Design review of the part built by this model. Coordinates are the model's own, in mm. A direction names the side the tool comes from. Give positions to 0.01 mm unless a question says otherwise; leave off trailing zeros. Loops run counter-clockwise (first coordinate to the right, second up) from the corner with the lowest first, then second, coordinate; pieces in that order, holes last. Notation, with made-up numbers: (0, 44.5) - (40, 44.5) arc R28 ccw to (40, 70.5) - close; hole circle Ø5 at (12, 43). An arc over 180 degrees is marked (long way). One line per item, written item: value. Start each with the question number.
```python
from build123d import *

# Parameters (mm, degrees)
SKETCH1_R                       = 13
BOSS_EXTRUDE1_DEPTH             = 28
SKETCH3_R                       = 24
BOSS_EXTRUDE2_DEPTH             = 1
SKETCH2_R                       = 10
CUT_EXTRUDE1_DEPTH              = 1
CUT_EXTRUDE1_DEPTH_BACK         = 30
SKETCH9_R                       = 13
BOSS_EXTRUDE3_DEPTH             = 17.5
CHAMFER2_SIZE                   = 0.5
CHAMFER3_SIZE                   = 0.5
CHAMFER4_SIZE                   = 0.5
SKETCH11_R                      = 10
CUT_EXTRUDE5_DEPTH              = 1
CUT_EXTRUDE5_DEPTH_BACK         = 46.5
CHAMFER5_SIZE                   = 0.5
SKETCH7_R                       = 2.5
WYTNIJ_WYCI_GNI_CIE1_DEPTH      = 28
WYTNIJ_WYCI_GNI_CIE1_DEPTH_BACK = 19.5
WYTNIJ_WYCI_GNI_CIE2_DEPTH      = 10
ZAOKR_GLENIE1_R                 = 4
ZAOKR_GLENIE2_R                 = 1


with BuildPart() as part:
    # Sketch1 → Boss-Extrude1 (new body)
    with BuildSketch(Plane(origin=(0, 0, 0), x_dir=(1, 0, 0), z_dir=(0, 1, 0))):
        Circle(SKETCH1_R)
    extrude(amount=-BOSS_EXTRUDE1_DEPTH)

    # Sketch3 → Boss-Extrude2 (add, symmetric)
    with BuildSketch(Plane(origin=(0, 0, 0), x_dir=(1, 0, 0), z_dir=(0, 1, 0))):
        Circle(SKETCH3_R)
    extrude(amount=BOSS_EXTRUDE2_DEPTH, both=True)

    # Sketch2 → Cut-Extrude1 (cut, two sides)
    with BuildSketch(Plane(origin=(0, -28, 0), x_dir=(-1, 0, 0), z_dir=(0, -1, 0))) as cut_extrude1_sk:
        Circle(SKETCH2_R)
    extrude(amount=CUT_EXTRUDE1_DEPTH, mode=Mode.SUBTRACT)
    extrude(cut_extrude1_sk.sketch, amount=-CUT_EXTRUDE1_DEPTH_BACK, mode=Mode.SUBTRACT)

    # Sketch9 → Boss-Extrude3 (add)
    with BuildSketch(Plane(origin=(0, 0, 0), x_dir=(1, 0, 0), z_dir=(0, 1, 0))):
        Circle(SKETCH9_R)
    extrude(amount=BOSS_EXTRUDE3_DEPTH)

    # Chamfer2
    chamfer2_edges = [part.edges().sort_by_distance(p)[0] for p in [
        (-24, -1, 0),
    ]]
    chamfer(chamfer2_edges, length=CHAMFER2_SIZE)

    # Chamfer3
    chamfer3_edges = [part.edges().sort_by_distance(p)[0] for p in [
        (-24, 1, 0),
    ]]
    chamfer(chamfer3_edges, length=CHAMFER3_SIZE)

    # Chamfer4
    chamfer4_edges = [part.edges().sort_by_distance(p)[0] for p in [
        (-13, -28, 0),
    ]]
    chamfer(chamfer4_edges, length=CHAMFER4_SIZE)

    # Sketch11 → Cut-Extrude5 (cut, two sides)
    with BuildSketch(Plane(origin=(0, 17.5, 0), x_dir=(1, 0, 0), z_dir=(0, 1, 0))) as cut_extrude5_sk:
        Circle(SKETCH11_R)
    extrude(amount=CUT_EXTRUDE5_DEPTH, mode=Mode.SUBTRACT)
    extrude(cut_extrude5_sk.sketch, amount=-CUT_EXTRUDE5_DEPTH_BACK, mode=Mode.SUBTRACT)

    # Chamfer5
    chamfer5_edges = [part.edges().sort_by_distance(p)[0] for p in [
        (-13, 17.5, 0),
    ]]
    chamfer(chamfer5_edges, length=CHAMFER5_SIZE)

    # Sketch7 → Wytnij-wyciągnięcie1 (cut, two sides)
    with BuildSketch(Plane.XZ.offset(1)) as wytnij_wyci_gni_cie1_sk:
        with Locations((0, 19)):
            Circle(SKETCH7_R)
        with Locations((3.299315376, -18.711347307)):
            Circle(SKETCH7_R)
        with Locations((-6.497936067, 17.852932618)):
            Circle(SKETCH7_R)
        with Locations((9.5, 16.454482672)):
            Circle(SKETCH7_R)
        with Locations((-19, 0)):
            Circle(SKETCH7_R)
        with Locations((-8.029746973, -17.219847954)):
            Circle(SKETCH7_R)
        with Locations((-12.212964584, 14.554844419)):
            Circle(SKETCH7_R)
        with Locations((-14.575405337, -12.230217242)):
            Circle(SKETCH7_R)
        with Locations((-16.454482672, 9.5)):
            Circle(SKETCH7_R)
    extrude(amount=WYTNIJ_WYCI_GNI_CIE1_DEPTH, mode=Mode.SUBTRACT)
    extrude(wytnij_wyci_gni_cie1_sk.sketch, amount=-WYTNIJ_WYCI_GNI_CIE1_DEPTH_BACK, mode=Mode.SUBTRACT)

    # Szkic1 → Wytnij-wyciągnięcie2 (cut)
    with BuildSketch(Plane(origin=(0, 1, 0), x_dir=(1, 0, 0), z_dir=(0, 1, 0))):
        with BuildLine():
            Line((13.831592317, -13.026398351), (17.289813207, -16.645190274))
            ThreePointArc((17.289813207, -16.645190274), (23.635386072, 4.167556264), (10.554119522, 21.554826863))
            Line((10.554119522, 21.554826863), (8.542154603, 16.971493592))
            ThreePointArc((8.542154603, 16.971493592), (18.711347307, 3.299315376), (13.831592317, -13.026398351))
        make_face()
    extrude(amount=-WYTNIJ_WYCI_GNI_CIE2_DEPTH, mode=Mode.SUBTRACT)

    # Zaokrąglenie1
    zaokr_glenie1_edges = [part.edges().sort_by_distance(p)[0] for p in [
        (13.831592317, 0, 13.026398351),
        (8.542154603, 0, -16.971493592),
    ]]
    fillet(zaokr_glenie1_edges, radius=ZAOKR_GLENIE1_R)

    # Zaokrąglenie2
    zaokr_glenie2_edges = [part.edges().sort_by_distance(p)[0] for p in [
        (10.554119522, 0, -21.554826863),
        (17.289813207, 0, 16.645190274),
    ]]
    fillet(zaokr_glenie2_edges, radius=ZAOKR_GLENIE2_R)


solid = part.part
```
(1) Draft analysis for pull direction X (two halves, no side actions). For faces 1 (the cylindrical face through (-10.316, -14.064, 7.91)), 2 (the cylindrical face through (-0.66, -5.57, -9.98)), 3 (the cylindrical face through (16.877, -0.014, 16.466)), state which applies: pulls with the +X half, pulls with the -X half, needs draft (parallel to the pull), parting line crosses it, or undercut.
(2) Take a section at C-C on y = -19. State the section outline as (x, z) points.
(3) Take a section at A-A on x = 0. State the section outline as (y, z) points.
(4) Take a section at D-D on x = -7. State how many separate pieces and enclosed holes the cut face has, and give its area (3 significant figures).
(5) For pin 1 Ø3 at (x, y) = (-10.5, -15) entering from +Z; pin 2 Ø8 at (x, z) = (7, 4.5) entering from -Y; pin 3 Ø1 at (y, z) = (-18, -11.5) entering from +X; pin 4 Ø6 at (x, z) = (-6.5, 17.85) entering from +Y, all flat-tipped, find the tip position at first contact; note any pin that passes through.
(6) Take a section at B-B on z = 0. State the section outline as (x, y) points.
(7) Machinability: for faces 4 (the flat face through (-12, -1, -6)), 5 (the cylindrical face through (-0.33, -0.01, 21.48)), which of the approach directions +Z, -Z, +X, -X, +Y, -Y give a long, thin tool a straight path to every point of the face, cutting with its end or side? Answer none if there is none.
(8) To check wall thickness, follow L1, parallel to Z at x = -4.5, y = 0; L2, parallel to Y at x = -1, z = -16; L3, parallel to X at y = -13, z = -4.5. State the ranges of each line that lie inside material, in increasing order. Write a range as from..to.
Here are the results:
1. face 1: parting line crosses it
1. face 2: undercut
1. face 3: pulls with the +X half
2. outline: circle Ø26 at (0, 0); hole circle Ø20 at (0, 0)
3. outline: (-28, -12.5) - (-27.5, -13) - (-1, -13) - (-1, -23.5) - (-0.5, -24) - (0.5, -24) - (1, -23.5) - (1, -13) - (17, -13) - (17.5, -12.5) - (17.5, -10) - (-28, -10) - close; (-28, 10) - (17.5, 10) - (17.5, 12.5) - (17, 13) - (1, 13) - (1, 16.5) - (-1, 16.5) - (-1, 13) - (-27.5, 13) - (-28, 12.5) - close; (-1, 21.5) - (1, 21.5) - (1, 23.5) - (0.5, 24) - (-0.5, 24) - (-1, 23.5) - close
4. separate pieces: 4
4. enclosed holes: 0
4. area: 375 mm²
5. pin 1: z = 9.38
5. pin 2: y = -28
5. pin 3: x = 6.93
5. pin 4: y = 1
6. outline: (-24, -0.5) - (-23.5, -1) - (-21.5, -1) - (-21.5, 1) - (-23.5, 1) - (-24, 0.5) - close; (-16.5, -1) - (-13, -1) - (-13, -27.5) - (-12.5, -28) - (-10, -28) - (-10, 17.5) - (-12.5, 17.5) - (-13, 17) - (-13, 1) - (-16.5, 1) - close; (10, -28) - (12.5, -28) - (13, -27.5) - (13, -1) - (19, -1) - (19, 1) - (13, 1) - (13, 17) - (12.5, 17.5) - (10, 17.5) - close
7. face 4: -Y
7. face 5: +Y, -Y
8. L1: -23.57..-8.93, 8.93..16.35, 19.36..23.57
8. L2: -1..1
8. L3: -12.2..-8.93, 8.93..12.2
